```python
from build123d import *

# Parameters (mm, degrees)
SKETCH_1_R          = 56
EXTRUDE_1_DEPTH     = 27
SKETCH_3_R          = 29.5
EXTRUDE_2_DEPTH     = 5
FILLET_1_R          = 5
SKETCH_6_R          = 7.5
CUT_EXTRUDE_1_DEPTH = 33
FILLET_2_R          = 1
FILLET_3_R          = 1


with BuildPart() as part:
    # Эскиз1 → Бобышка-Вытянуть1 (new body)
    with BuildSketch(Plane(origin=(0, 0, 0), x_dir=(1, 0, 0), z_dir=(0, 1, 0))):
        with Locations(Location((0, 0, 0), (0, 0, 270))):
            Circle(SKETCH_1_R)
    extrude(amount=-EXTRUDE_1_DEPTH)

    # Эскиз3 → Бобышка-Вытянуть2 (add)
    with BuildSketch(Plane(origin=(0, -27, 0), x_dir=(-1, 0, 0), z_dir=(0, -1, 0))):
        with Locations(Location((0, 0, 0), (0, 0, 270))):
            Circle(SKETCH_3_R)
    extrude(amount=EXTRUDE_2_DEPTH)

    # Скругление1
    fillet_1_edges = [part.edges().sort_by_distance(p)[0] for p in [
        (0, -32, -29.5),
    ]]
    fillet(fillet_1_edges, radius=FILLET_1_R - 0.0001)  # a hair under: the kernel refuses the full size

    # Эскиз6 → Вырез-Вытянуть1 (cut)
    with BuildSketch(Plane.XZ.offset(32)):
        with Locations(Location((0, 0, 0), (0, 0, 270))):
            Circle(SKETCH_6_R)
    extrude(amount=-CUT_EXTRUDE_1_DEPTH, mode=Mode.SUBTRACT)

    # Скругление2
    fillet_2_edges = [part.edges().sort_by_distance(p)[0] for p in [
        (0, -32, 7.5),
    ]]
    fillet(fillet_2_edges, radius=FILLET_2_R)

    # Скругление3
    fillet_3_edges = [part.edges().sort_by_distance(p)[0] for p in [
        (0, 0, -56),
        (0, -27, -56),
    ]]
    fillet(fillet_3_edges, radius=FILLET_3_R)


solid = part.part
```
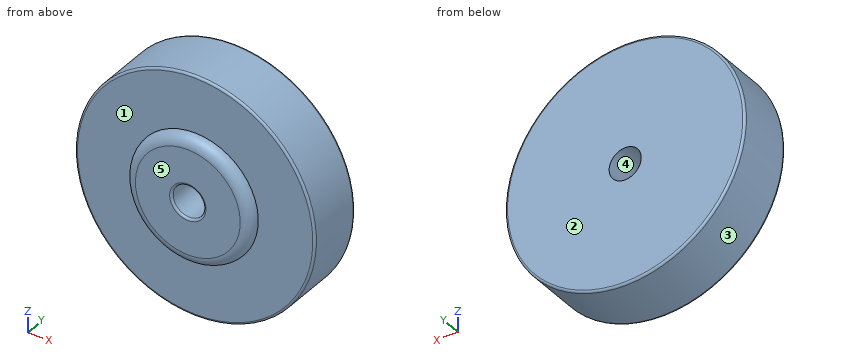
For this review, take the finished solid that the model builds, in its own axes (mm). Face numbers are marked on the shaded views. A direction names the side the tool comes from. Give positions to 0.01 mm unless a question says otherwise; leave off trailing zeros. Write each loop counter-clockwise with the first axis right and the second up, starting at its lowest first coordinate (ties: lowest second). Pieces come first, ordered by that corner, then holes.
Item 1: Wall thickness on probe 1 along X at (y, z) = (-18, 0); probe 2 along Y at (x, z) = (-11.5, -30); probe 3 along Z at (x, y) = (21, -10.5): over which ranges is each line inside the solid? List them lowest first.
Item 2: Insertion check: P1, Ø5, axis at y = -4, z = -7.5, coming from the +X side; P2, Ø6, axis at y = -17, z = -44.5, coming from the -X side; P3, Ø1, axis at x = -42, z = 35, coming from the -Y side; P4, Ø12, axis at x = 0, z = 0, coming from the +Y side. Each pin has a flat end and moves straight along its axis. Give the tip position at first contact, or say it passes through.
Item 3: Take a section at C-C (y = -20.5). Give the boundary of the cut face in (x, z), and give its area (3 significant figures).
Item 4: Machinability: for the marked faces 1 and 2, which of the approach directions +Z, -Z, +X, -X, +Y, -Y give a long, thin tool a straight path to every point of the face, cutting with its end or side? Answer none if there is none.
Item 5: The part is to be moulded in two halves that separate along X. For the marked faces 3, 4 and 5, say which applies: +X half, -X half, draft (parallel to the pull), parting line (faces both ways), or undercut.
Established:
1. probe 1: x = -56 to -7.5, 7.5 to 56
1. probe 2: y = -27 to 0
1. probe 3: z = -51.91 to 51.91
2. P1: stops at x = 55.78
2. P2: stops at x = -37.6
2. P3: stops at y = -27
2. P4: passes through
3. outline: circle Ø112 at (0, 0); hole circle Ø15 at (0, 0)
3. area: 9,680 mm2
4. face 1: -Y
4. face 2: +Z, -Z, +X, -X, +Y
5. face 3: parting line
5. face 4: undercut
5. face 5: draft
